from build123d import *

# Parameters (mm, degrees)
SKETCH_R     = 5.75
PAD_DEPTH    = 5
SKETCH001_R  = 2.9
PAD001_DEPTH = 5
SKETCH002_W  = 11.5
SKETCH002_H  = 23
PAD002_DEPTH = 23.5
SKETCH003_W  = 11.5
SKETCH003_H  = 32
PAD003_DEPTH = 4.5
SKETCH004_R  = 2
POCKET_DEPTH = 23.501


with BuildPart() as part:
    # Sketch → Pad (new body)
    with BuildSketch(Plane.XY):
        Circle(SKETCH_R)
    extrude(amount=PAD_DEPTH)

    # Sketch001 → Pad001 (join)
    with BuildSketch(Plane.XY):
        with Locations((0, -6.35)):
            Circle(SKETCH001_R)
    extrude(amount=PAD001_DEPTH)

    # Sketch002 → Pad002 (join)
    with BuildSketch(Plane.XY):
        with Locations((0, -5.75)):
            Rectangle(SKETCH002_W, SKETCH002_H)
    extrude(amount=-PAD002_DEPTH)

    # Sketch003 → Pad003 (join)
    with BuildSketch(Plane.XY):
        with Locations((0, -5.75)):
            Rectangle(SKETCH003_W, SKETCH003_H)
    extrude(amount=-PAD003_DEPTH)

    # Sketch004 → Pocket (cut, through all)
    with BuildSketch(Plane.XY):
        with Locations((0, 8.25)):
            Circle(SKETCH004_R)
        with Locations((0, -19.75)):
            Circle(SKETCH004_R)
    extrude(amount=-POCKET_DEPTH, mode=Mode.SUBTRACT)


with BuildPart() as part_1:
    # Body placement: moved
    add(part.part.moved(Location((0, 0, -1))))


solid = part_1.part
Input: part model. Units: mm. Frame: model coordinates. A direction names the side the tool comes from. Give positions to 0.01 mm unless a question says otherwise; leave off trailing zeros. Order: outer loops, then holes, each group sorted by start corner. A loop starts at its lowest first (then second) coordinate and runs counter-clockwise, first axis right, second up. Notation, with made-up numbers: M -19.75,-22 L 12.25,-22 A4 ccw 12.25,-17 Z; hole C 48,19 d7. An arc over 180 degrees is marked long. Answer as a JSON object with one key per item and string values.
1. Ray query, line 1 (X direction, y = 8.25, z = -3.1); line 2 (Z direction, x = 4.5, y = -15); line 3 (Z direction, x = -3.5, y = 7). Return the intervals inside material, ascending. Write a range as [from, to].
Result sheet:
{"line 1": "[-5.75, -2], [2, 5.75]", "line 2": "[-24.5, -1]", "line 3": "[-5.5, -1]"}
2. First-contact query: P1, Ø5, axis at y = 6.5, z = -6, coming from the +X side; P2, Ø1, axis at x = -1, z = -15.5, coming from the +Y side; P3, Ø5, axis at x = -1, y = -18.5, coming from the +Z side; P4, Ø5, axis at x = -1, y = 9, coming from the -Z side. Flat tips, straight axial feed; report the tip coordinate or a pass-through.
Result sheet:
{"P1": "x = 5.75", "P2": "y = 5.75", "P3": "z = -1", "P4": "z = -5.5"}
3. Cut plane C-C, the plane z = -13.5. Output: boundary loops of the cut face in (x, y), and give its area (4 significant figures).
Result sheet:
{"outline": "M -5.75,-17.25 L 5.75,-17.25 L 5.75,5.75 L -5.75,5.75 Z", "area": "264.5 mm²"}
4. Cut plane B-B, the plane x = 1.25. Output: boundary loops of the cut face in (y, z).
Result sheet:
{"outline": "M -21.75,-5.5 L -21.31,-5.5 L -21.31,-1 L -21.75,-1 Z; M -18.19,-5.5 L -17.25,-5.5 L -17.25,-24.5 L 5.75,-24.5 L 5.75,-5.5 L 6.69,-5.5 L 6.69,-1 L 5.61,-1 L 5.61,4 L -8.97,4 L -8.97,-1 L -18.19,-1 Z; M 9.81,-5.5 L 10.25,-5.5 L 10.25,-1 L 9.81,-1 Z"}
5. Cut plane A-A, the plane y = -19. Output: boundary loops of the cut face in (x, z).
Result sheet:
{"outline": "M -5.75,-5.5 L -1.85,-5.5 L -1.85,-1 L -5.75,-1 Z; M 1.85,-5.5 L 5.75,-5.5 L 5.75,-1 L 1.85,-1 Z"}
6. Cut plane D-D, the plane y = -6.35. Output: boundary loops of the cut face in (x, z), and give its area (3 significant figures).
Result sheet:
{"outline": "M -5.75,-24.5 L 5.75,-24.5 L 5.75,-1 L 2.9,-1 L 2.9,4 L -2.9,4 L -2.9,-1 L -5.75,-1 Z", "area": "299 mm²"}
7. Reachability of faces 1 (the flat face through (-1.4, 6.5, -5.5)), 2 (the flat face through (0, -17.25, -15)), 3 (the cylindrical face through (-0.08, -9.25, 1.46)) from +Z, -Z, +X, -X, +Y, -Y: full face, straight path, thin tool, end or side. Return the list, or none.
Result sheet:
{"face 1": "-Z, +X, -X, +Y", "face 2": "-Z, +X, -X, -Y", "face 3": "+Z"}
